The listing builds one solid part. Answer for the finished solid, in the listing's coordinates (mm). Face numbers are marked on the shaded views. Coordinates: 2 decimals unless noted, no trailing zeros. Answer as a JSON object with one key per item and string values. Group by question number.
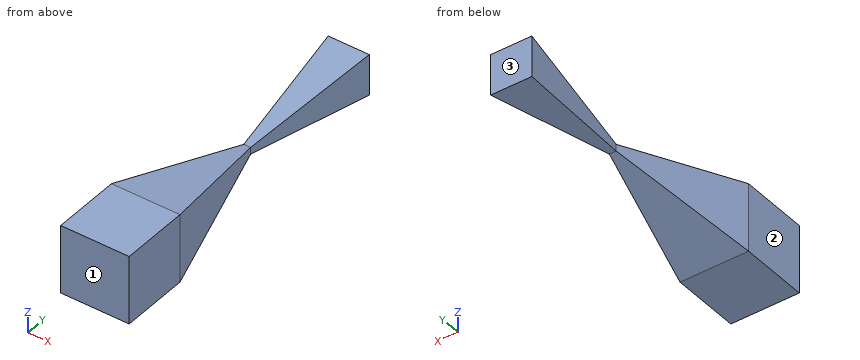
from build123d import *

# Parameters (mm, degrees)
F2_W      = 500
F2_H      = 500
F1_W      = 50
F1_H      = 50
F5_W      = 300
F5_H      = 300
F3_FACE_W = 500
F3_FACE_H = 500
F7_DEPTH  = 500


with BuildPart() as f3:
    # F2 (on offset) → F3 section 0
    with BuildSketch(Plane.XZ.offset(1000)):
        Rectangle(F2_W, F2_H)
    # F1 (on Front) → F3 section 1
    with BuildSketch(Plane.XZ):
        Rectangle(F1_W, F1_H)
    loft()

    # F1 (on Front) → F6 section 0
    with BuildSketch(Plane.XZ):
        Rectangle(F1_W, F1_H)
    # F5 (on offset) → F6 section 1
    with BuildSketch(Plane.XZ.offset(-1000)):
        Rectangle(F5_W, F5_H)
    loft()

    # F3_face (on face) → F7 (join)
    with BuildSketch(Plane.XZ.offset(1000)):
        Rectangle(F3_FACE_W, F3_FACE_H)
    extrude(amount=F7_DEPTH)


solid = f3.part
Item 1: Flat-ended cylindrical pins translate along their axes: pin 1 Ø4 at (y, z) = (323.5, -35) entering from -X; pin 2 Ø2 at (y, z) = (603, -53.5) entering from -X; pin 3 Ø2 at (y, z) = (-861, -175) entering from -X. Find the tip coordinate at first contact, or state that the pin passes through.
Item 2: Consider L1, parallel to X at y = -600, z = -153; L2, parallel to Z at x = 154, y = -623 (3 decimals); L3, parallel to X at y = 149.5, z = 39. Determine where each line is inside the solid, lowest interval first. Write a range as from..to.
Item 3: For a pull along Y with two mould halves and no side action, classify the marked faces 1, 2 and 3 as +Y half, -Y half, draft (parallel to the pull), parting line (faces both ways), or undercut.
Answer:
{
 "1": {"pin 1": "x = -65.69", "pin 2": "x = -100.5", "pin 3": "x = -218.95"},
 "2": {"L1": "-160..160", "L2": "-165.175..165.175", "L3": "-43.69..43.69"},
 "3": {"face 1": "-Y half", "face 2": "draft", "face 3": "+Y half"}
}
